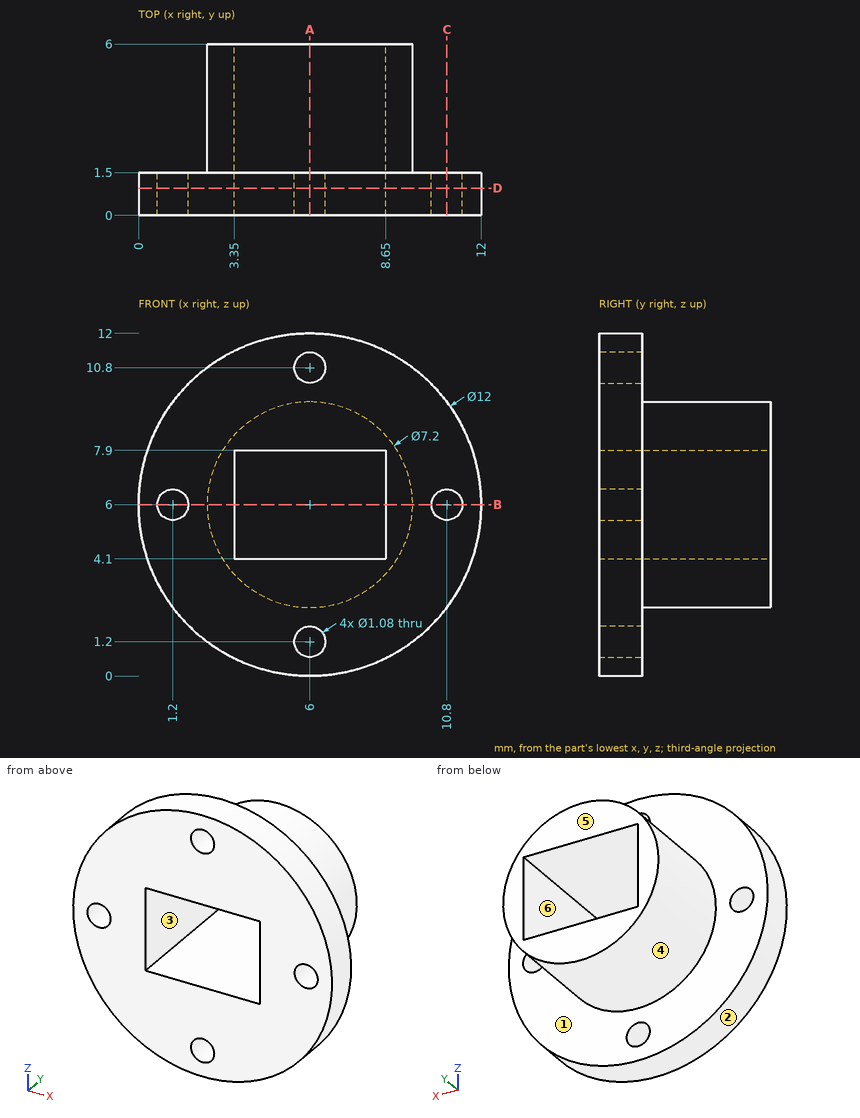
Check sheet for the drawn part. Datum: minimum x, y, z corner. Units: mm. A direction names the side the tool comes from. Round coordinates to 2 decimals unless told otherwise and drop trailing zeros. Write each loop counter-clockwise with the first axis right and the second up, starting at its lowest first coordinate (ties: lowest second). Pieces come first, ordered by that corner, then holes. Notation, with made-up numbers: (29, 56) -> (72, 56) arc R15 ccw to (72, 68) -> close; hole circle Ø11 at (35.5, 48.5). An arc over 180 degrees is marked (long way). Write each question's results on one line, items separated by ' | '. Start each with the question number.
1. Cross-section at A-A (x = 6). Enter the section's corners in (y, z), then the cut area to 3 significant figures.
2. Draft check along X on the marked faces 1, 2 and 3. Enter one of: +X half, -X half, draft (parallel to the pull), parting line (faces both ways), or undercut.
3. Cross-section at C-C (x = 10.8). Enter the section's corners in (y, z).
4. Cross-section at D-D (y = 0.95). Enter the section's corners in (x, z).
5. Material ranges on probe 1 along X at (y, z) = (0.6, 1.2); probe 2 along Y at (x, z) = (3, 2); probe 3 along X at (y, z) = (5.65, 5.25), recorded low to high. Write a range as from..to.
6. Set-up check for the marked faces 4, 5 and 6: record each of +Z, -Z, +X, -X, +Y, -Y from which the full face is reachable in a straight line by a thin tool's end or side.
7. Depth check by flat-ended pin: P1, Ø1.2, axis at x = 6, z = 10.8, coming from the -Y side; P2, Ø1.1, axis at y = 4.5, z = 6.5, coming from the -X side; P3, Ø1.6, axis at x = 5, y = 2, coming from the -Z side; P4, Ø2, axis at y = 4, z = 7, coming from the +X side. Enter the tip coordinate at first touch or a pass-through.
8. Cross-section at B-B (z = 6). Enter the section's corners in (x, y).
Solutions:
1) outline: (0, 0) -> (1.5, 0) -> (1.5, 0.66) -> (0, 0.66) -> close; (0, 1.74) -> (1.5, 1.74) -> (1.5, 2.4) -> (6, 2.4) -> (6, 4.1) -> (0, 4.1) -> close; (0, 7.9) -> (6, 7.9) -> (6, 9.6) -> (1.5, 9.6) -> (1.5, 10.26) -> (0, 10.26) -> close; (0, 11.34) -> (1.5, 11.34) -> (1.5, 12) -> (0, 12) -> close | area: 24.4 mm2
2) face 1: draft | face 2: parting line | face 3: undercut
3) outline: (0, 2.4) -> (1.5, 2.4) -> (1.5, 5.46) -> (0, 5.46) -> close; (0, 6.54) -> (1.5, 6.54) -> (1.5, 9.6) -> (0, 9.6) -> close
4) outline: circle Ø12 at (6, 6); hole circle Ø1.08 at (1.2, 6); hole (3.35, 4.1) -> (8.65, 4.1) -> (8.65, 7.9) -> (3.35, 7.9) -> close; hole circle Ø1.08 at (6, 1.2); hole circle Ø1.08 at (6, 10.8); hole circle Ø1.08 at (10.8, 6)
5) probe 1: x = 2.4..5.46, 6.54..9.6 | probe 2: y = 0..1.5 | probe 3: x = 2.48..3.35, 8.65..9.52
6) face 4: +Y | face 5: +Z, -Z, +X, -X, +Y | face 6: +Y, -Y
7) P1: stops at y = 0 | P2: stops at x = 2.4 | P3: stops at z = 0.01 | P4: stops at x = 9.6
8) outline: (0, 0) -> (0.66, 0) -> (0.66, 1.5) -> (0, 1.5) -> close; (1.74, 0) -> (3.35, 0) -> (3.35, 6) -> (2.4, 6) -> (2.4, 1.5) -> (1.74, 1.5) -> close; (8.65, 0) -> (10.26, 0) -> (10.26, 1.5) -> (9.6, 1.5) -> (9.6, 6) -> (8.65, 6) -> close; (11.34, 0) -> (12, 0) -> (12, 1.5) -> (11.34, 1.5) -> close
